Part model, mm, in its own coordinate system. Face numbers are marked on the shaded views. A direction names the side the tool comes from. Give positions to 0.01 mm unless a question says otherwise; leave off trailing zeros. Write each loop counter-clockwise with the first axis right and the second up, starting at its lowest first coordinate (ties: lowest second). Pieces come first, ordered by that corner, then holes. Notation, with made-up numbers: (-21.75, 54) - (-11.75, 54) arc R25 ccw to (-11.75, 81) - close; hole circle Ø8 at (42.25, 0.5). An arc over 180 degrees is marked (long way). Answer as a JSON object with one key per item and string values. Group by question number.
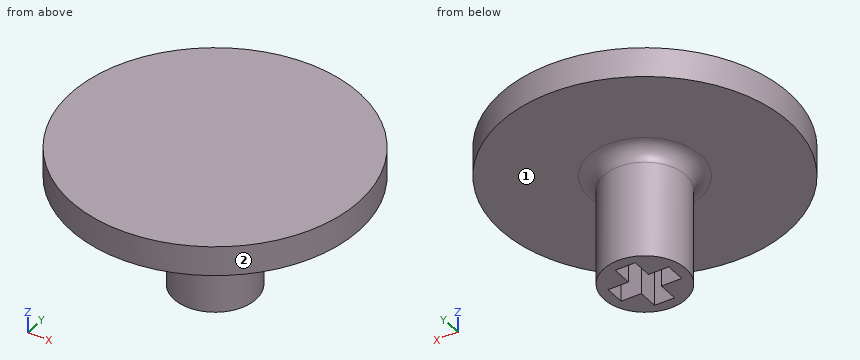
```python
from build123d import *

# Parameters (mm, degrees)
F0_W     = 2.77
F0_H     = 7.5
F3_DEPTH = 7.5
F4_R     = 1


with BuildPart() as f1:
    # F0 (on Front) → F1 (revolve)
    with BuildSketch(Plane.XZ):
        Polygon((0, 9.5), (0, 7.5), (2.77, 7.5), (9.75, 7.5), (9.75, 9.5), align=None)
        with Locations((1.385, 3.75)):
            Rectangle(F0_W, F0_H)
    revolve(axis=Axis((0, 0, 3.75), (0, 0, 1)))

    # F2 (on face) → F3 (cut)
    with BuildSketch(Plane(origin=(0, 0, 0), x_dir=(1, 0, 0), z_dir=(0, 0, -1))):
        Polygon((0.675, 2.05), (-0.675, 2.05), (-0.675, 0.675), (-2.05, 0.675), (-2.05, -0.675), (-0.675, -0.675), (-0.675, -2.05), (0.675, -2.05), (0.675, -0.675), (2.05, -0.675), (2.05, 0.675), (0.675, 0.675), align=None)
    extrude(amount=-F3_DEPTH, mode=Mode.SUBTRACT)

    # F4
    f4_edges = [f1.edges().sort_by_distance(p)[0] for p in [
        (-2.77, 0, 7.5),
    ]]
    fillet(f4_edges, radius=F4_R)


solid = f1.part
```
1) Band-saw the part on D-D (x = 8). List the corners of the cut face in (y, z), plus the area to 3 significant figures.
2) Drop flat-ended pins along their axis: P1, Ø1.5, axis at x = 0, z = 4.5, coming from the +Y side; P2, Ø0.7, axis at y = -1, z = 4.5, coming from the +X side; P3, Ø5, axis at y = 7.5, z = 6, coming from the +X side. Give the stop position or say it passes through.
3) Band-saw the part on B-B (x = 0). List the corners of the cut face in (y, z).
4) Which spindle directions (+Z, -Z, +X, -X, +Y, -Y) get a long thin tool onto all of the face, cutting with end or side? Do the marked faces 1 and 2. Say none if no direction does.
5) Probe line 1 (Z direction, x = -1.5, y = -5.5); line 2 (Y direction, x = -1.5, z = 4) (3 decimals); line 3 (Y direction, x = -1.75, z = 1.5) (3 decimals). List the from-to ranges inside material, lowest first.
6) Band-saw the part on A-A (z = 2.5). List the corners of the cut face in (x, y) (3 decimals), plus the area to 3 significant figures.
Verdict:
{
 "1": {"outline": "(-5.57, 7.5) - (5.57, 7.5) - (5.57, 9.5) - (-5.57, 9.5) - close", "area": "22.3 mm2"},
 "2": {"P1": "y = 2.77", "P2": "x = 2.69", "P3": "x = 8.05"},
 "3": {"outline": "(-9.75, 7.5) - (-3.77, 7.5) arc R1 cw to (-2.77, 6.5) - (-2.77, 0) - (-2.05, 0) - (-2.05, 7.5) - (2.05, 7.5) - (2.05, 0) - (2.77, 0) - (2.77, 6.5) arc R1 cw to (3.77, 7.5) - (9.75, 7.5) - (9.75, 9.5) - (-9.75, 9.5) - close"},
 "4": {"face 1": "-Z", "face 2": "+Z, -Z"},
 "5": {"line 1": "7.5 to 9.5", "line 2": "-2.329 to -0.675, 0.675 to 2.329", "line 3": "-2.147 to -0.675, 0.675 to 2.147"},
 "6": {"outline": "circle Ø5.54 at (0, 0); hole (-2.05, -0.675) - (-0.675, -0.675) - (-0.675, -2.05) - (0.675, -2.05) - (0.675, -0.675) - (2.05, -0.675) - (2.05, 0.675) - (0.675, 0.675) - (0.675, 2.05) - (-0.675, 2.05) - (-0.675, 0.675) - (-2.05, 0.675) - close", "area": "14.9 mm2"}
}
